Build history of the part. All positions in model axes, mm. Face numbers are marked on the shaded views. A direction names the side the tool comes from. Give positions to 0.01 mm unless a question says otherwise; leave off trailing zeros. Write each loop counter-clockwise with the first axis right and the second up, starting at its lowest first coordinate (ties: lowest second). Pieces come first, ordered by that corner, then holes. Notation, with made-up numbers: M -3,22.25 L 49,22.25 A24 cw 49,42.25 Z; hole C 17.5,45 d10. An arc over 180 degrees is marked long. Return JSON: item names as keys, results as strings. Group by question number.
Q1. Tool access for the marked faces 5, 6, 7, 8 and 9: list every direction of +Z, -Z, +X, -X, +Y, -Y with a clear straight run to the whole face (end or side of a thin tool).
Q2. Band-saw the part on A-A, the plane x = 31.5. Give the cut face in (y, z), then the cut area to 3 significant figures.
Q3. Band-saw the part on D-D, the plane z = 8. Count the separate pieces of the cut face and the enclosed holes in it, then the cut area to 3 significant figures.
Q4. Band-saw the part on B-B, the plane y = 24.5. Give the cut face in (x, z), then the cut area to 3 significant figures.
Q5. Pull direction Y, two halves, no side cores. Call the marked faces 1, 2, 3 and 4: +Y half, -Y half, draft (parallel to the pull), parting line (faces both ways), or undercut.
Q6. Flat gauge pins, fed straight in: pin 1 Ø7.5 at (x, z) = (-43.5, 14) entering from +Y; pin 2 Ø22.5 at (x, y) = (-45, 45) entering from -Z; pin 3 Ø2 at (y, z) = (51.5, 17) entering from +X; pin 4 Ø8 at (x, z) = (-5, 9.5) entering from +Y. Where does each tip first touch, or does it go through?
Q7. Wall check: probe 1 along X at (y, z) = (-15.5, 8.75); probe 2 along Y at (x, z) = (-55, 8); probe 3 along Y at (x, z) = (-38, 22). Give the ranges that are in metal, low to high.
Q8. Band-saw the part on C-C, the plane y = 41.5. Give the cut face in (x, z), then the cut area to 3 significant figures.
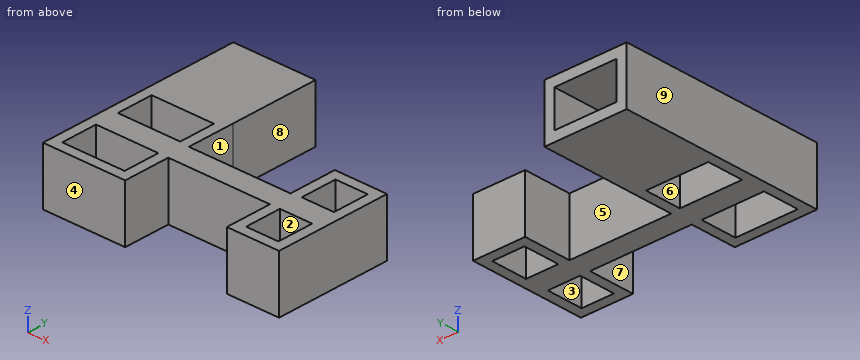
Autodesk Inventor part; units mm, degrees
ref_plane "YZ Plane" through (0, 0, 0) normal (1, 0, 0) x (0, 1, 0)
ref_plane "XZ Plane" through (0, 0, 0) normal (0, 1, 0) x (-1, 0, 0)
ref_plane "XY Plane" through (0, 0, 0) normal (0, 0, 1) x (1, 0, 0)
sketch "Sketch1" plane through (0, 0, 0) normal (0, 0, 1) x (1, 0, 0)
  line L0 (-60.2002, 26.1718) -> (-60.2002, -26.2038) construction
  line L1 (-60.2002, -26.2038) -> (-23, -26.2038) construction
  line L2 (-23, -26.2038) -> (-23, -5.3034) construction
  line L3 (23, -5.3034) -> (-23, -5.3034) construction
  line L4 (23, -5.3034) -> (23, -26.2034) construction
  line L5 (23, -26.2034) -> (46.6, -26.2034) construction
  line L6 (46.6, -26.2034) -> (46.6, 26.2034) construction
  line L7 (23, 26.2034) -> (46.6, 26.2034) construction
  line L8 (23, 11.4966) -> (23, 26.2034) construction
  line L9 (-8.3, 4.6966) -> (8.3, 4.6966) construction
  line L10 (-23.0002, 26.1718) -> (-23.0002, 11.4966) construction
  line L11 (-23.0002, 26.1718) -> (-60.2002, 26.1718) construction
  line L12 (-27.5, -5.3034) -> (-55.7, -5.3034) construction
  line L13 (-27.5, -5.3034) -> (-27.5, -21.7034) construction
  line L14 (-27.5, -21.7034) -> (-55.7, -21.7034) construction
  line L15 (-55.7, -21.7034) -> (-55.7, -5.3034) construction
  line L16 (42.1, -5.3034) -> (27.5, -5.3034) construction
  line L17 (42.1, -5.3034) -> (42.1, -21.7034) construction
  line L18 (42.1, -21.7034) -> (27.5, -21.7034) construction
  line L19 (27.5, -21.7034) -> (27.5, -5.3034) construction
  line L20 (42.1, 5.3034) -> (42.1, 21.7034) construction
  line L21 (27.5, 5.3034) -> (42.1, 5.3034) construction
  line L22 (27.5, 21.7034) -> (27.5, 5.3034) construction
  line L23 (42.1, 21.7034) -> (27.5, 21.7034) construction
  line L24 (-55.7, 21.7034) -> (-55.7, 5.3034) construction
  line L25 (-27.5, 21.7034) -> (-55.7, 21.7034) construction
  line L26 (-27.5, 5.3034) -> (-27.5, 21.7034) construction
  line L27 (-55.7, 5.3034) -> (-27.5, 5.3034) construction
  line L28 (-60.2002, 26.1718) -> (-23, 26.1718)
  line L29 (-23, -26.2038) -> (-60.2002, -26.2038)
  line L30 (-60.2002, -26.2038) -> (-60.2002, 26.1718)
  line L31 (-55.7, 21.7034) -> (-27.5, 21.7034)
  line L32 (-27.5, 21.7034) -> (-27.5, 5.3034)
  line L33 (-27.5, 5.3034) -> (-55.7, 5.3034)
  line L34 (-55.7, 5.3034) -> (-55.7, 21.7034)
  line L35 (-55.7, -5.3034) -> (-27.5, -5.3034)
  line L36 (-27.5, -5.3034) -> (-27.5, -21.7034)
  line L37 (-27.5, -21.7034) -> (-55.7, -21.7034)
  line L38 (-55.7, -21.7034) -> (-55.7, -5.3034)
  line L39 (-23, 4.6966) -> (23, 4.6966)
  line L40 (23, 26.2034) -> (46.6, 26.2034)
  line L41 (46.6, 26.2034) -> (46.6, -26.2034)
  line L42 (46.6, -26.2034) -> (23, -26.2034)
  line L43 (27.5, 21.7034) -> (42.1, 21.7034)
  line L44 (42.1, 21.7034) -> (42.1, 5.3034)
  line L45 (42.1, 5.3034) -> (27.5, 5.3034)
  line L46 (27.5, 5.3034) -> (27.5, 21.7034)
  line L47 (27.5, -5.3034) -> (42.1, -5.3034)
  line L48 (42.1, -5.3034) -> (42.1, -21.7034)
  line L49 (42.1, -21.7034) -> (27.5, -21.7034)
  line L50 (27.5, -21.7034) -> (27.5, -5.3034)
  line L51 (-23, -5.3034) -> (23, -5.3034)
  line L52 (-23, 26.1718) -> (-23, 4.6966)
  line L53 (-23, -5.3034) -> (-23, -26.2038)
  line L54 (23, -26.2034) -> (23, -5.3034)
  line L55 (23, 4.6966) -> (23, 26.2034)
  point P0 (0, 0)
  point P1 (0, 0)
  point P2 (0, 0)
extrude "Extrusion1" add sketch "Sketch1" along normal blind 25.4
sketch "Sketch2" plane through (-60.2002, 26.1718, 0) normal (0, 1, 0) x (1, 0, 0)
  line L0 (4.5, -4.5) -> (32.7, -4.5)
  line L1 (32.7, -4.5) -> (32.7, -20.9)
  line L2 (32.7, -20.9) -> (4.5, -20.9)
  line L3 (4.5, -20.9) -> (4.5, -4.5)
  line L4 (37.2, 0) -> (0, 0)
  line L5 (0, 0) -> (0, -25.4)
  line L6 (0, -25.4) -> (37.2, -25.4)
  line L7 (37.2, -25.4) -> (37.2, 0)
  line L8 (0, 0) -> (37.2002, 0) construction
  dimension "d2" = 4.5
extrude "Extrusion2" add sketch "Sketch2" along normal blind 40
properties part number "mid_front_Chasis"
From the geometry:
{
 "1": {"face 5": "+Z, -Z, +Y", "face 6": "+Z, -Z", "face 7": "+Z, -Z, -Y", "face 8": "+Z, -Z, +X, +Y", "face 9": "+Z, -Z, -X, +Y, -Y"},
 "2": {"outline": "M -26.2,0 L -21.7,0 L -21.7,25.4 L -26.2,25.4 Z; M -5.3,0 L 5.3,0 L 5.3,25.4 L -5.3,25.4 Z; M 21.7,0 L 26.2,0 L 26.2,25.4 L 21.7,25.4 Z", "area": "498 mm^2"},
 "3": {"separate pieces": "1", "enclosed holes": "4", "area": "2,600 mm^2"},
 "4": {"outline": "M -60.2,0 L -23,0 L -23,25.4 L -60.2,25.4 Z; M 23,0 L 46.6,0 L 46.6,25.4 L 23,25.4 Z", "area": "1,540 mm^2"},
 "5": {"face 1": "draft", "face 2": "undercut", "face 3": "undercut", "face 4": "-Y half"},
 "6": {"pin 1": "stops at y = 26.17", "pin 2": "stops at z = 0", "pin 3": "stops at x = -23", "pin 4": "stops at y = 4.7"},
 "7": {"probe 1": "x = -60.2 to -55.7, -27.5 to -23, 23 to 27.5, 42.1 to 46.6", "probe 2": "y = -26.2 to -21.7, -5.3 to 5.3, 21.7 to 26.17", "probe 3": "y = -26.2 to -21.7, -5.3 to 5.3, 21.7 to 66.17"},
 "8": {"outline": "M -60.2,0 L -23,0 L -23,25.4 L -60.2,25.4 Z; hole M -55.7,4.5 L -27.5,4.5 L -27.5,20.9 L -55.7,20.9 Z", "area": "482 mm^2"}
}
